```python
from build123d import *

# Parameters (mm, degrees)
SKETCH1_R           = 4.572
BOSS_EXTRUDE1_DEPTH = 66.04
SKETCH3_W           = 2.286
SKETCH3_H           = 2.286
BOSS_EXTRUDE3_DEPTH = 12.7


with BuildPart() as part:
    # Sketch1 → Boss-Extrude1 (new body)
    with BuildSketch(Plane.XY):
        Circle(SKETCH1_R)
    extrude(amount=BOSS_EXTRUDE1_DEPTH)

    # Sketch3 → Boss-Extrude3 (add)
    with BuildSketch(Plane(origin=(0, 0, 0), x_dir=(-1, 0, 0), z_dir=(0, 0, -1))):
        with Locations((0, 4.426819965)):
            Rectangle(SKETCH3_W, SKETCH3_H)
    extrude(amount=-BOSS_EXTRUDE3_DEPTH)


solid = part.part
```
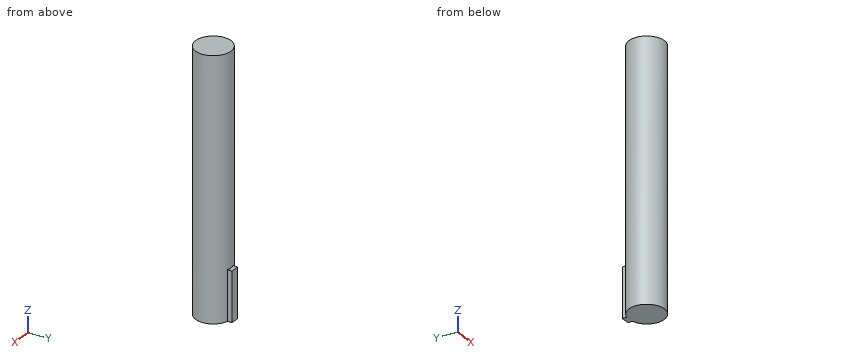
Here's how the part is built. I have some questions about the finished solid (model axes, mm). Round coordinates to 2 decimals unless told otherwise and drop trailing zeros. Loops run counter-clockwise (first coordinate to the right, second up) from the corner with the lowest first, then second, coordinate; pieces in that order, holes last. Notation, with made-up numbers: (28.5, 59.25) -> (34.5, 59.25) arc R21 ccw to (34.5, 92.25) -> close; hole circle Ø2 at (8, 54). An arc over 180 degrees is marked (long way). Answer as CSV lines item,"result". Start each with the question number.
1. I'm going to push flat-ended pins straight in: P1, Ø1, axis at y = 1, z = 30, coming from the +X side; P2, Ø2, axis at x = 2.5, z = 19, coming from the +Y side. Where does each tip first touch, or does it pass through?
2. Imagine slicing it at A-A on x = 0. Write out the boundary of the cut face in (y, z).
3. Imagine slicing it at D-D on z = 11.5. Write out the boundary of the cut face in (x, y), plus the area to 3 significant figures.
4. Imagine slicing it at B-B on z = 30. Write out the boundary of the cut face in (x, y).
5. I need wall thicknesses on probe 1 along Y at (x, z) = (0, 16); probe 2 along Z at (x, y) = (0, 4.75); probe 3 along X at (y, z) = (3.25, 21). Which ranges of each line are inside material? Lowest first, please. Write a range as from..to.
6. Imagine slicing it at C-C on y = 2.5. Write out the boundary of the cut face in (x, z).
Solution:
1,P1,"x = 4.54"
1,P2,"y = 4.32"
2,outline,"(-4.57, 0) -> (5.57, 0) -> (5.57, 12.7) -> (4.57, 12.7) -> (4.57, 66.04) -> (-4.57, 66.04) -> close"
3,outline,"(-1.14, 4.43) arc R4.57 ccw (long way) to (1.14, 4.43) -> (1.14, 5.57) -> (-1.14, 5.57) -> close"
3,area,"68.1 mm²"
4,outline,"circle Ø9.14 at (0, 0)"
5,probe 1,"-4.57..4.57"
5,probe 2,"0..12.7"
5,probe 3,"-3.22..3.22"
6,outline,"(-3.83, 0) -> (3.83, 0) -> (3.83, 66.04) -> (-3.83, 66.04) -> close"
